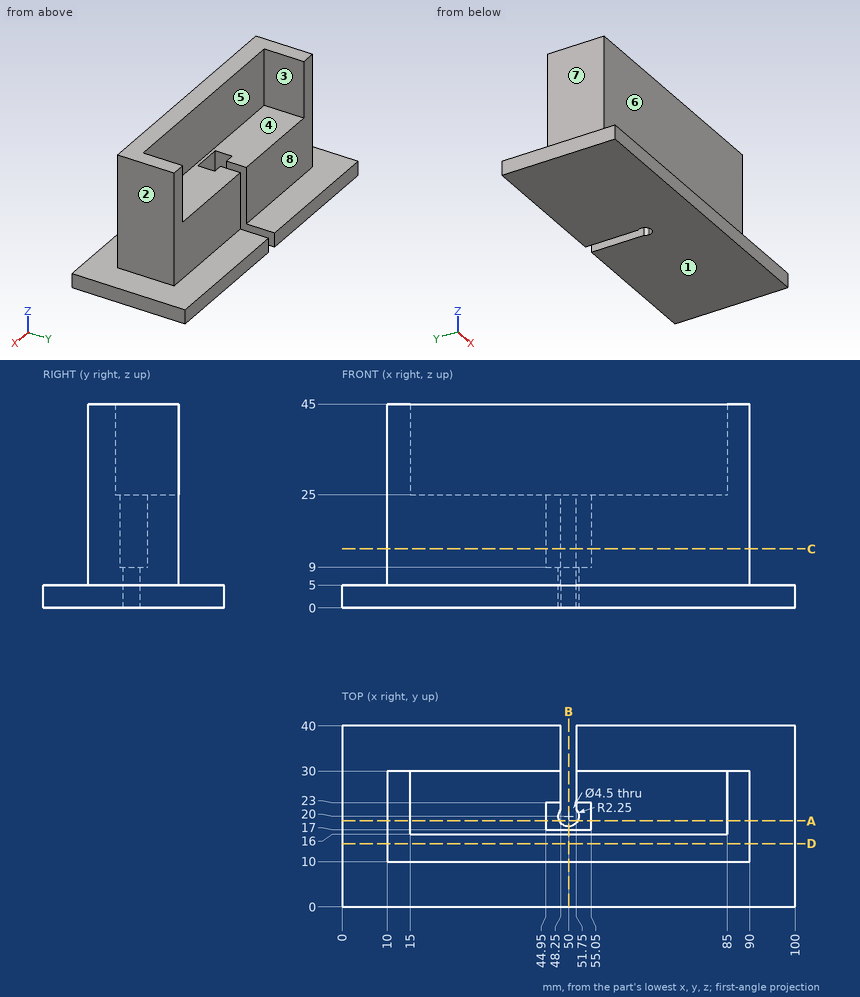
Study the drawing (mm; zero at the part's minimum x, y, z) and answer. A direction names the side the tool comes from. Coordinates: 2 decimals unless noted, no trailing zeros. Write each loop counter-clockwise with the first axis right and the second up, starting at its lowest first coordinate (ties: lowest second). Pieces come first, ordered by that corner, then holes.
Q1. A cutting plane is placed at A-A, the plane y = 19. Give the vertices of the cut face in (x, z).
Q2. Determine the mould class of the marked faces 1, 2, 3 and 4 for opening direction X: released by +X, released by -X, zero draft, split by the parting line, or undercut.
Q3. Find the intervals of material crossed by line 1 (X direction, y = 23.5, z = 23); line 2 (X direction, y = 20, z = 2); line 3 (Z direction, x = 65, y = 23), in increasing order.
Q4. A cutting plane is placed at C-C, the plane z = 13. Give the vertices of the cut face in (x, y).
Q5. A cutting plane is placed at B-B, the plane x = 50. Give the vertices of the cut face in (y, z), then the cut area to 3 significant figures.
Q6. A cutting plane is placed at D-D, the plane y = 14. Give the vertices of the cut face in (x, z), then the cut area to 3 significant figures.
Q7. Which of the six approach directions +Z, -Z, +X, -X, +Y, -Y give full straight-line access (tool end or side, diameter ignored) to the marked faces 5, 6, 7 and 8?
Q8. Each of these flat-tipped pins is pushed along its axis until it touches: pin 1 Ø8 at (x, z) = (46.5, 6) entering from +Y; pin 2 Ø6 at (x, y) = (30, 34) entering from +Z; pin 3 Ø5 at (y, z) = (31, 37.5) entering from +X; pin 4 Ø3 at (x, z) = (52.5, 14) entering from +Y. Where does it stop, or does it pass through?
Findings below:
1. outline: (0, 0) - (47.98, 0) - (47.98, 9) - (44.95, 9) - (44.95, 25) - (15, 25) - (15, 45) - (10, 45) - (10, 5) - (0, 5) - close; (52.02, 0) - (100, 0) - (100, 5) - (90, 5) - (90, 45) - (85, 45) - (85, 25) - (55.05, 25) - (55.05, 9) - (52.02, 9) - close
2. face 1: zero draft
2. face 2: released by +X
2. face 3: undercut
2. face 4: undercut
3. line 1: x = 10 to 48.25, 51.75 to 90
3. line 2: x = 0 to 47.75, 52.25 to 100
3. line 3: z = 0 to 25
4. outline: (10, 10) - (90, 10) - (90, 30) - (51.75, 30) - (51.75, 23) - (55.05, 23) - (55.05, 17) - (44.95, 17) - (44.95, 23) - (48.25, 23) - (48.25, 30) - (10, 30) - close
5. outline: (0, 0) - (17.75, 0) - (17.75, 9) - (17, 9) - (17, 25) - (16, 25) - (16, 45) - (10, 45) - (10, 5) - (0, 5) - close
5. area: 352 mm2
6. outline: (0, 0) - (100, 0) - (100, 5) - (90, 5) - (90, 45) - (10, 45) - (10, 5) - (0, 5) - close
6. area: 3,700 mm2
7. face 5: +Z, +Y
7. face 6: +Z, +X, -X, -Y
7. face 7: +Z, -X, +Y, -Y
7. face 8: +Z, +X, -X, +Y
8. pin 1: stops at y = 40
8. pin 2: stops at z = 5
8. pin 3: stops at x = 90
8. pin 4: stops at y = 30
